Design review of the part built by this model. Coordinates are the model's own, in mm. Coordinates: 2 decimals unless noted, no trailing zeros. Write each loop counter-clockwise with the first axis right and the second up, starting at its lowest first coordinate (ties: lowest second). Pieces come first, ordered by that corner, then holes.
Q1. Take a section at B-B (z = -4.25). Give the boundary of the cut face in (x, y), and give its area (3 significant figures).
Q2. Take a section at A-A (x = 7). Give the boundary of the cut face in (y, z), and give its area (3 significant figures).
Q3. For probe 1 along Z at (x, y) = (22, 0.75); probe 2 along X at (y, z) = (2, 9); probe 3 along X at (y, z) = (1.7, -9), list the stretches that pass through material, from the lowest coordinate up.
Q4. Take a section at C-C (y = 1.15). Give the boundary of the cut face in (x, z).
Q5. Take a section at D-D (x = 21.5). Give the boundary of the cut face in (y, z), and give its area (3 significant figures).
```python
from build123d import *

# Parameters (mm, degrees)
PERFIL_PRINCIPAL_W           = 50
PERFIL_PRINCIPAL_H           = 25
BASE_DEPTH                   = 3
PERFIL_CORTE_W               = 23
PERFIL_CORTE_H               = 12.4
CORTE_PRINCIPAL_DEPTH        = 82.921801368
ESBO_O7_W                    = 12
ESBO_O7_H                    = 3
ESBO_O7_W_2                  = 17.5
CORTE_EXTRUS_O3_DEPTH        = 91.332942436
FURO_DE_DI_METRO_3_0_3_1_D   = 3
FURO_DE_DI_METRO_2_6_2_6_1_D = 2.6
FILETE1_R                    = 3


with BuildPart() as part:
    # Perfil Principal → Base (new body)
    with BuildSketch(Plane(origin=(0, 0, 0), x_dir=(1, 0, 0), z_dir=(0, 1, 0))):
        Rectangle(PERFIL_PRINCIPAL_W, PERFIL_PRINCIPAL_H)
    extrude(amount=BASE_DEPTH)

    # Perfil Corte → Corte Principal (cut, through all)
    with BuildSketch(Plane(origin=(49.188016516, 0, 22.11675526), x_dir=(-1, 0, 0), z_dir=(0, -1, 0))):
        with Locations((57.368016516, 22.11675526)):
            Rectangle(PERFIL_CORTE_W, PERFIL_CORTE_H)
    extrude(amount=-CORTE_PRINCIPAL_DEPTH, mode=Mode.SUBTRACT)

    # Esboço7 → Corte-extrusão3 (cut, through all)
    with BuildSketch(Plane(origin=(56.452995871, 0, 26.44162237), x_dir=(-1, 0, 0), z_dir=(0, -1, 0))):
        with Locations((64.632995871, 34.14162237)):
            Rectangle(ESBO_O7_W, ESBO_O7_H)
        with Locations((64.632995871, 18.74162237)):
            Rectangle(ESBO_O7_W_2, ESBO_O7_H)
    extrude(amount=-CORTE_EXTRUS_O3_DEPTH, mode=Mode.SUBTRACT)

    # Furo de diâmetro Ø3.0 (3)1 (through all)
    with Locations(Plane(origin=(0, 3, 0), x_dir=(1, 0, 0), z_dir=(0, 1, 0))):
        with Locations((22, 9), (22, -9)):
            Hole(FURO_DE_DI_METRO_3_0_3_1_D / 2)

    # Furo de diâmetro Ø2.6 (2.6)1 (through all)
    with Locations(Plane(origin=(0, 3, 0), x_dir=(1, 0, 0), z_dir=(0, 1, 0))):
        with Locations((-22, 9), (-22, -9), (7, 9), (7, -9)):
            Hole(FURO_DE_DI_METRO_2_6_2_6_1_D / 2)

    # Filete1
    filete1_edges = [part.edges().sort_by_distance(p)[0] for p in [
        (-25, 1.5, 12.5),
        (-25, 1.5, -12.5),
        (25, 1.5, -12.5),
        (25, 1.5, 12.5),
    ]]
    fillet(filete1_edges, radius=FILETE1_R)


solid = part.part
```
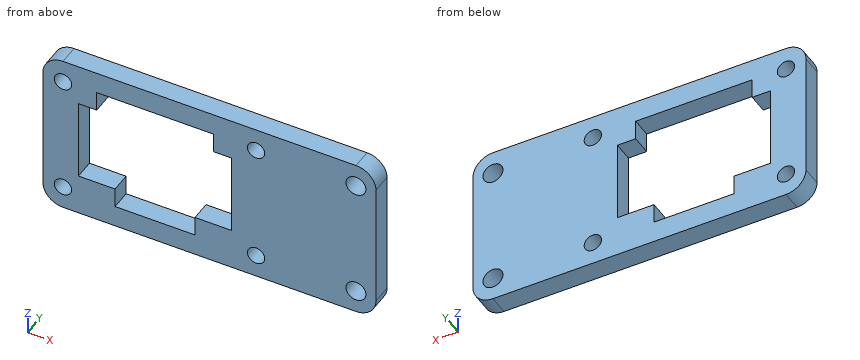
Response:
1. outline: (-25, 0) - (-19.68, 0) - (-19.68, 3) - (-25, 3) - close; (3.32, 0) - (25, 0) - (25, 3) - (3.32, 3) - close
1. area: 81.0 mm2
2. outline: (0, -12.5) - (3, -12.5) - (3, -10.3) - (0, -10.3) - close; (0, -7.7) - (3, -7.7) - (3, 7.7) - (0, 7.7) - close; (0, 10.3) - (3, 10.3) - (3, 12.5) - (0, 12.5) - close
2. area: 59.4 mm2
3. probe 1: z = -12.5 to -10.5, -7.5 to 7.5, 10.5 to 12.5
3. probe 2: x = -25 to -23.3, -20.7 to -16.93, 0.57 to 5.7, 8.3 to 20.5, 23.5 to 25
3. probe 3: x = -25 to -23.3, -20.7 to -14.18, -2.18 to 5.7, 8.3 to 20.5, 23.5 to 25
4. outline: (-25, -9.5) arc R3 ccw to (-22, -12.5) - (22, -12.5) arc R3 ccw to (25, -9.5) - (25, 9.5) arc R3 ccw to (22, 12.5) - (-22, 12.5) arc R3 ccw to (-25, 9.5) - close; hole circle Ø2.6 at (-22, -9); hole circle Ø2.6 at (-22, 9); hole (-19.68, -6.2) - (-14.18, -6.2) - (-14.18, -9.2) - (-2.18, -9.2) - (-2.18, -6.2) - (3.32, -6.2) - (3.32, 6.2) - (0.57, 6.2) - (0.57, 9.2) - (-16.93, 9.2) - (-16.93, 6.2) - (-19.68, 6.2) - close; hole circle Ø2.6 at (7, -9); hole circle Ø2.6 at (7, 9); hole circle Ø3 at (22, -9); hole circle Ø3 at (22, 9)
5. outline: (0, -12.5) - (3, -12.5) - (3, -10.41) - (0, -10.41) - close; (0, -7.59) - (3, -7.59) - (3, 7.59) - (0, 7.59) - close; (0, 10.41) - (3, 10.41) - (3, 12.5) - (0, 12.5) - close
5. area: 58.0 mm2
